```python
from build123d import *

# Parameters (mm, degrees)
CUT_EXTRUDE1_DEPTH  = 3.3
BOSS_EXTRUDE1_DEPTH = 14.3


with BuildPart() as part:
    # Sketch1 → Revolve1 (revolve)
    with BuildSketch(Plane(origin=(0, 0, 0), x_dir=(0, 0, -1), z_dir=(1, 0, 0))):
        Polygon((-7, 0), (-7, 2.8), (-6.8, 3), (138.15, 3), (138.15, 0), align=None)
    revolve(axis=Axis((0, 0, -138.15), (0, 0, 1)))

    # Sketch2 → Cut-Revolve1 (revolve, cut)
    with BuildSketch(Plane(origin=(0, 0, 0), x_dir=(0, 0, -1), z_dir=(1, 0, 0))):
        Polygon((-7, 0), (-7, 2.05), (-6.6, 1.65), (-5.5, 1.65), (-5.5, 1.5), (-5.2295, 1.2295), (4, 1.2295), (4.709852156, 0), align=None)
    revolve(axis=Axis((0, 0, -4.709852156), (0, 0, 1)), mode=Mode.SUBTRACT)

    # Sketch3 → Cut-Extrude1 (cut)
    with BuildSketch(Plane.XY.offset(4.3)):
        Polygon((-6.447248163, -4.742941189), (3.2120101, -7.33113164), (5.800200551, 2.328126623), (3.385385985, 2.975174236), (1.12071934, -5.476676744), (-3.708909791, -4.182581519), (-1.444243147, 4.269269461), (-3.859057712, 4.916317074), align=None)
    extrude(amount=CUT_EXTRUDE1_DEPTH, mode=Mode.SUBTRACT)

    # Sketch4 → Boss-Extrude1 (add)
    with BuildSketch(Plane.XY.offset(-138.15)):
        with BuildLine():
            Line((4.5, -4.5), (4.5, 4.5))
            ThreePointArc((4.5, 4.5), (3.181980515, 7.681980515), (0, 9))
            ThreePointArc((0, 9), (-3.181980515, 7.681980515), (-4.5, 4.5))
            Line((-4.5, 4.5), (-4.5, -4.5))
            ThreePointArc((-4.5, -4.5), (-3.181980515, -7.681980515), (0, -9))
            ThreePointArc((0, -9), (3.181980515, -7.681980515), (4.5, -4.5))
        make_face()
    extrude(amount=BOSS_EXTRUDE1_DEPTH)


solid = part.part
```
Build history of the part. All positions in model axes, mm. A direction names the side the tool comes from. Coordinates: 2 decimals unless noted, no trailing zeros. Order: outer loops, then holes, each group sorted by start corner. A loop starts at its lowest first (then second) coordinate and runs counter-clockwise, first axis right, second up.
Item 1: Drill centre lines: L1, parallel to Y at x = 0, z = -0.25; L2, parallel to Y at x = 0, z = 6.25; L3, parallel to Y at x = 1.25, z = -43. Where is each one in solid material? Low to high.
Filled in:
L1: y = -3 to -1.23, 1.23 to 3
L2: y = -3 to -1.65, 1.65 to 3
L3: y = -2.73 to 2.73
Item 2: Saw through at B-B on y = 6.25. List the corners of the cut face in (x, z), then the cut area to 3 significant figures.
Filled in:
outline: (-4.15, -138.15) - (4.15, -138.15) - (4.15, -123.85) - (-4.15, -123.85) - close
area: 119 mm2
Item 3: Mould opens along Y. For faces 1 (the cylindrical face through (0.748, -0.976, 0.55)), 2 (the cylindrical face through (0, -3, -59)), 3 (the flat face through (-3, -2, -123.85)), 4 (the conical face through (-0.059, 0.187, -4.597)) say: released by +Y, released by -Y, zero draft, split by the parting line, or undercut.
Filled in:
face 1: undercut
face 2: split by the parting line
face 3: zero draft
face 4: undercut
Item 4: Drop flat-ended pins along their axis: pin 1 Ø6 at (y, z) = (0.5, -14.5) entering from -X; pin 2 Ø4 at (y, z) = (-3.5, -13) entering from +X; pin 3 Ø1.5 at (x, y) = (1, -0.5) entering from +Z; pin 4 Ø0.5 at (x, y) = (-2.5, 1) entering from +Z. Give the stop position or say it passes through.
Filled in:
pin 1: stops at x = -3
pin 2: stops at x = 2.6
pin 3: stops at z = 6.82
pin 4: stops at z = 7
Item 5: Saw through at A-A on z = -61.5. List the corners of the cut face in (x, y), then the cut area to 3 significant figures.
Filled in:
outline: circle Ø6 at (0, 0)
area: 28.3 mm2
Item 6: Tool access for faces 5 (the flat face through (-2.42, 0.62, 5.63)), 6 (the cylindrical face through (-1.115, -1.216, 6.042)), 7 (the flat face through (0, 0, -138.15)), 8 (the flat face through (2.42, -0.62, 5.63)): list every direction of +Z, -Z, +X, -X, +Y, -Y with a clear straight run to the whole face (end or side of a thin tool).
Filled in:
face 5: +Z, -X, +Y
face 6: +Z
face 7: -Z, +X, -X, +Y, -Y
face 8: +Z, +X, -Y
